from build123d import *

# Parameters (mm, degrees)
F1_DEPTH = 4
F2_R     = 10
F3_R     = 1
F4_R     = 2
F5_R     = 1


with BuildPart() as f1:
    # F0 (on Top) → F1 (new body)
    with BuildSketch(Plane.XY):
        with BuildLine():
            Line((-4.5, 0.4868329805), (-4.5, 9.4868329805))
            ThreePointArc((-4.5, 9.4868329805), (-10.4641425726, 0.8670180042), (-6, -8.6168439698))
            Line((-6, -8.6168439698), (6, -8.6168439698))
            ThreePointArc((6, -8.6168439698), (10.4641425726, 0.8670180042), (4.5, 9.4868329805))
            Line((4.5, 9.4868329805), (4.5, 0.4868329805))
            ThreePointArc((4.5, 0.4868329805), (0, -1.5131670195), (-4.5, 0.4868329805))
        make_face()
        with BuildLine():
            Line((6, -8.6168439698), (-6, -8.6168439698))
            ThreePointArc((-6, -8.6168439698), (0, -10.5), (6, -8.6168439698))
        make_face()
        with BuildLine():
            ThreePointArc((6, -8.6168439698), (0, -10.5), (-6, -8.6168439698))
            Line((-6, -8.6168439698), (-6, -38.6168439698))
            Line((-6, -38.6168439698), (6, -38.6168439698))
            Line((6, -38.6168439698), (6, -8.6168439698))
        make_face()
    extrude(amount=F1_DEPTH)

    # F2
    f2_edges = [f1.edges().sort_by_distance(p)[0] for p in [
        (-6, -8.616844, 2),
        (6, -8.616844, 2),
    ]]
    fillet(f2_edges, radius=F2_R)

    # F3
    f3_edges = [f1.edges().sort_by_distance(p)[0] for p in [
        (-4.5, 9.486833, 2),
        (4.5, 9.486833, 2),
    ]]
    fillet(f3_edges, radius=F3_R)

    # F4
    f4_edges = [f1.edges().sort_by_distance(p)[0] for p in [
        (6, -38.616844, 2),
        (-6, -38.616844, 2),
    ]]
    fillet(f4_edges, radius=F4_R)

    # F5
    f5_edges = [f1.edges().sort_by_distance(p)[0] for p in [
        (4.5, 0.486833, 2),
        (-4.5, 0.486833, 2),
    ]]
    fillet(f5_edges, radius=F5_R)


solid = f1.part
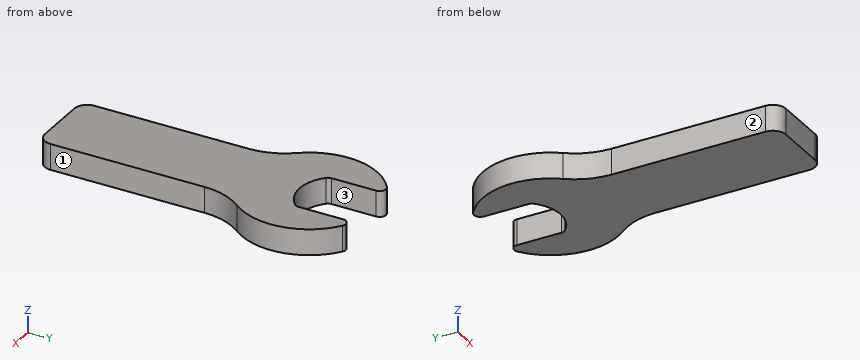
Part model, mm, in its own coordinate system. Face numbers are marked on the shaded views. A direction names the side the tool comes from. Coordinates: 2 decimals unless noted, no trailing zeros. Order: outer loops, then holes, each group sorted by start corner. A loop starts at its lowest first (then second) coordinate and runs counter-clockwise, first axis right, second up.
(1) Pin check, flat tips, straight feed: pin 1 Ø2 at (y, z) = (4, 2.5) entering from -X; pin 2 Ø1.2 at (y, z) = (-20, 1.5) entering from -X. Stop position of each tip, or through.
Check sheet entries:
pin 1: stops at x = -10.06
pin 2: stops at x = -6
(2) Slice it at B-B, the plane z = 2.75. Write the cut outline in (x, y) (1 decimal).
Check sheet entries:
outline: (-8.2, -6.6) arc R10 cw to (-6, -12.8) - (-6, -36.6) arc R2 ccw to (-4, -38.6) - (4, -38.6) arc R2 ccw to (6, -36.6) - (6, -12.8) arc R10 cw to (8.2, -6.6) arc R10.5 ccw to (6.1, 8.6) arc R1 ccw to (4.5, 7.7) - (4.5, 0.9) arc R1 cw to (4.2, 0.2) arc R6.1 cw to (-4.2, 0.2) arc R1 cw to (-4.5, 0.9) - (-4.5, 7.7) arc R1 ccw to (-6.1, 8.6) arc R10.5 ccw to start
(3) Slice it at D-D, the plane y = -24. Write the cut outline in (x, z), and give its area (3 significant figures).
Check sheet entries:
outline: (-6, 0) - (6, 0) - (6, 4) - (-6, 4) - close
area: 48.0 mm2
(4) Probe L1, parallel to X at y = -26.5, z = 2.35; L2, parallel to X at y = 0.5, z = 3.65; L3, parallel to X at y = 6, z = 3.4. List the from-to ranges inside material, lowest first.
Check sheet entries:
L1: x = -6 to 6
L2: x = -10.49 to -4.42, 4.42 to 10.49
L3: x = -8.62 to -4.5, 4.5 to 8.62
(5) Tool access for the marked faces 1, 2 and 3: list every direction of +Z, -Z, +X, -X, +Y, -Y with a clear straight run to the whole face (end or side of a thin tool).
Check sheet entries:
face 1: +Z, -Z, +X, -Y
face 2: +Z, -Z, -X, -Y
face 3: +Z, -Z, +Y
(6) Slice it at A-A, the plane y = 1.5. Write the cut outline in (x, z), and give its area (3 significant figures).
Check sheet entries:
outline: (-10.39, 0) - (-4.5, 0) - (-4.5, 4) - (-10.39, 4) - close; (4.5, 0) - (10.39, 0) - (10.39, 4) - (4.5, 4) - close
area: 47.1 mm2
(7) Slice it at C-C, the plane x = -1. Write the cut outline in (y, z).
Check sheet entries:
outline: (-38.62, 0) - (-1.43, 0) - (-1.43, 4) - (-38.62, 4) - close
